Answer from the drawing. Dimensions are ordinates in mm from the lowest x, y and z of the part. Coordinates: 2 decimals unless noted, no trailing zeros. Order: outer loops, then holes, each group sorted by start corner. A loop starts at its lowest first (then second) coordinate and runs counter-clockwise, first axis right, second up. Notation, with made-up numbers: M -6,20.5 L 11,20.5 A12 ccw 11,40.5 Z; hole C 63.25,30.5 d1. An arc over 180 degrees is marked long. Use a Markdown table: item, result.
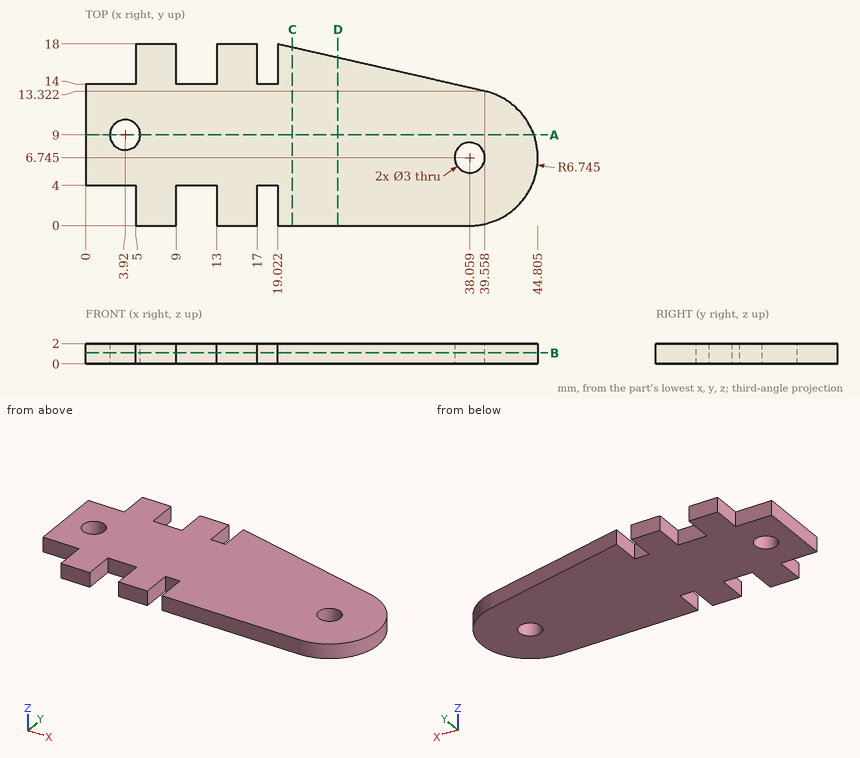
(1) Straight lines are drawn through the part: L1, parallel to Y at x = 4, z = 1.9; L2, parallel to Y at x = 18, z = 1.75; L3, parallel to X at y = 9.75, z = 1.25. For each, find the intervals that lie inside material, in ascending order.
Conclusion:
| item | result |
|---|---|
| L1 | 4 to 7.5, 10.5 to 14 |
| L2 | 4 to 14 |
| L3 | 0 to 2.62, 5.22 to 44.1 |
(2) Given P1, Ø0.6, axis at x = 2, z = 1, coming from the -Y side; P2, Ø10, axis at x = 12.5, y = 2.5, coming from the -Z side; P3, Ø0.6, axis at y = 15, z = 1, coming from the -X side, each flat-ended and moving along its own axis, determine where each tip first touches the part or whether it passes through.
Conclusion:
| item | result |
|---|---|
| P1 | y = 4 |
| P2 | z = 0 |
| P3 | x = 5 |
(3) A cutting plane is placed at A-A (y = 9). Determine the outline of the cut face in (x, z).
Conclusion:
| item | result |
|---|---|
| outline | M 0,0 L 2.42,0 L 2.42,2 L 0,2 Z; M 5.42,0 L 44.42,0 L 44.42,2 L 5.42,2 Z |
(4) A cutting plane is placed at B-B (z = 1.1). Determine the outline of the cut face in (x, y) (1 decimal), then the cut area to 3 significant figures.
Conclusion:
| item | result |
|---|---|
| outline | M 0,4 L 5,4 L 5,0 L 9,0 L 9,4 L 13,4 L 13,0 L 17,0 L 17,4 L 19,4 L 19,0 L 38.1,0 A6.7 ccw 39.6,13.3 L 19,18 L 19,14 L 17,14 L 17,18 L 13,18 L 13,14 L 9,14 L 9,18 L 5,18 L 5,14 L 0,14 Z; hole C 3.9,9 d3; hole C 38.1,6.7 d3 |
| area | 613 mm2 |
(5) A cutting plane is placed at C-C (x = 20.5). Determine the outline of the cut face in (y, z).
Conclusion:
| item | result |
|---|---|
| outline | M 0,0 L 17.66,0 L 17.66,2 L 0,2 Z |
(6) A cutting plane is placed at D-D (x = 25). Determine the outline of the cut face in (y, z).
Conclusion:
| item | result |
|---|---|
| outline | M 0,0 L 16.64,0 L 16.64,2 L 0,2 Z |
